Study the drawing (mm; zero at the part's minimum x, y, z) and answer. A direction names the side the tool comes from. Round coordinates to 2 decimals unless told otherwise and drop trailing zeros. Write each loop counter-clockwise with the first axis right and the second up, starting at its lowest first coordinate (ties: lowest second). Pieces come first, ordered by that corner, then holes.
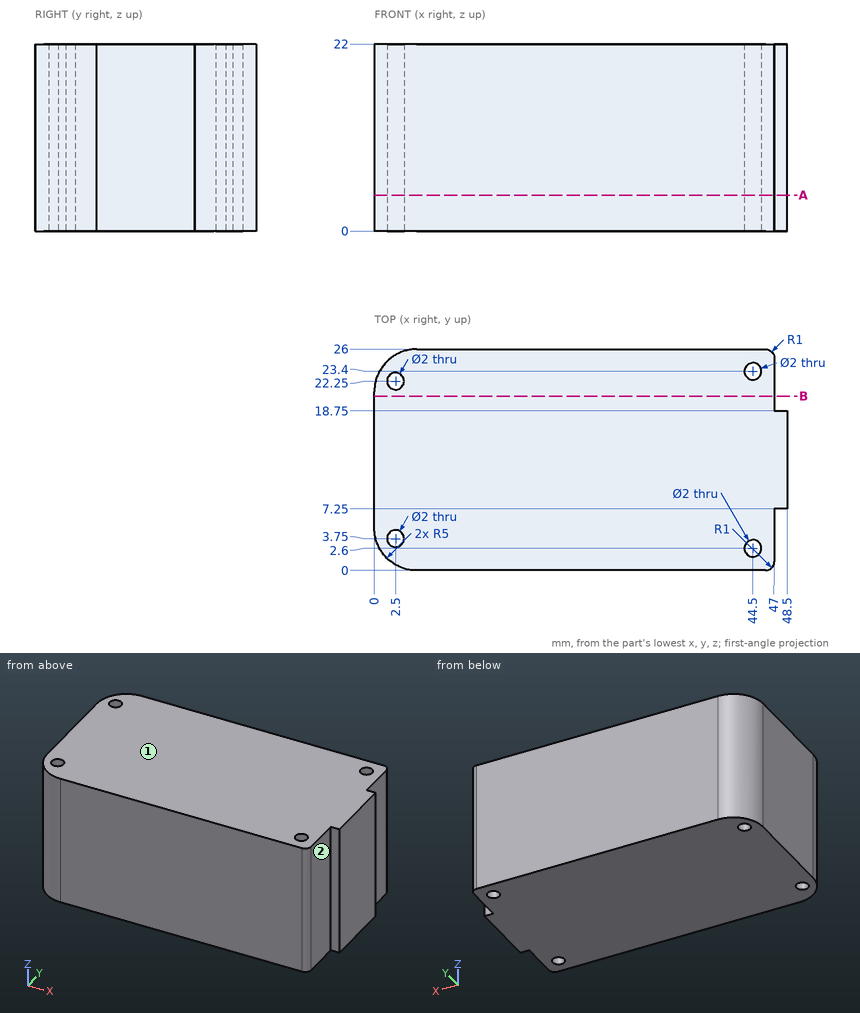
1. A tool of negligible diameter and unlimited length cuts with its end or side. For the marked faces 1 and 2, from which of +Z, -Z, +X, -X, +Y, -Y can it reach the whole face along a straight path? Write none if from no direction.
Geometry says:
face 1: +Z, +X, -X, +Y, -Y
face 2: +Z, -Z, +X, -Y
2. Straight lines are drawn through the part: line 1 along Y through (x, z) = (44.5, 11); line 2 along Y through (x, z) = (2.5, 15); line 3 along X through (y, z) = (2, 15). For each, find the intervals that lie inside material, in ascending order.
Geometry says:
line 1: y = 0 to 1.6, 3.6 to 22.4, 24.4 to 26
line 2: y = 0.67 to 2.75, 4.75 to 21.25, 23.25 to 25.33
line 3: x = 1 to 43.7, 45.3 to 47
3. Given pin 1 (1 mm diameter, centred on x = 10.5, z = 12, fed in from -Y); pin 2 (1.6 mm diameter, centred on x = 47.5, z = 11, fed in from +Y); pin 3 (1.9 mm diameter, centred on y = 20.5, z = 14, fed in from +X), each flat-ended and moving along its own axis, determine where each tip first touches the part or whether it passes through.
Geometry says:
pin 1: stops at y = 0
pin 2: stops at y = 25.71
pin 3: stops at x = 47
4. Section B-B on y = 20.5 is taken. Determine the outline of the cut face in (x, z).
Geometry says:
outline: (0, 0) - (47, 0) - (47, 22) - (0, 22) - close
5. Section A-A on z = 4.25 is taken. Determine the outline of the cut face in (x, y).
Geometry says:
outline: (0, 5) arc R5 ccw to (5, 0) - (46, 0) arc R1 ccw to (47, 1) - (47, 7.25) - (48.5, 7.25) - (48.5, 18.75) - (47, 18.75) - (47, 25) arc R1 ccw to (46, 26) - (5, 26) arc R5 ccw to (0, 21) - close; hole circle Ø2 at (2.5, 3.75); hole circle Ø2 at (2.5, 22.25); hole circle Ø2 at (44.5, 2.6); hole circle Ø2 at (44.5, 23.4)
